Can you work these out from the model? Positions are in its coordinate system, mm. A direction names the side the tool comes from. Round coordinates to 2 decimals unless told otherwise and drop trailing zeros. Loops run counter-clockwise (first coordinate to the right, second up) from the corner with the lowest first, then second, coordinate; pieces in that order, holes last.
(1) Will these pins go through, and if not, where does the flat tip stop? pin 1 Ø3 at (y, z) = (20.48, 18.5) entering from +X; pin 2 Ø8 at (x, y) = (16, -20) entering from +Z; pin 3 Ø6 at (x, y) = (-9.5, 18) entering from -Z; pin 4 Ø5 at (x, z) = (75, 31) entering from +Y.
(2) Which directions (+Z, -Z, +X, -X, +Y, -Y) give clear straight access to the entire face, cutting with the end or side of a thin tool? Please do faces 5 (the face through (-105, -6, 30)), 6 (the face through (1, -3, 13.5)), 7 (the face through (-109, -9, 21)).
(3) Thinking about a two-plate mould opening in Y: for faces 1 (the face through (-103, -9, 19)), 2 (the face through (103.289, 24.778, 6.844)), 3 (the face through (1, 30, 37)), 4 (the face through (-110.07, -21.896, 32.819)), which applies, released by +Y, released by -Y, zero draft, split by the parting line, or undercut?
(4) I want a section at A-A on x = -75. Write out the boundary of the cut face in (y, z).
(5) If I drill on line 1 along X through (y, z) = (15, 11); line 2 along Y through (x, z) = (-68, 4); line 3 along Z through (x, y) = (31.5, -19), over which ranges is the centre line in solid material (lowest first)?
(6) I want a section at C-C on x = 89. Write out the boundary of the cut face in (y, z), plus the area to 3 significant figures.
(7) I want a section at B-B on y = 8.5. Write out the boundary of the cut face in (x, z), plus the area to 3 significant figures.
from build123d import *

# Parameters (mm, degrees)
F0_W     = 115
F0_H     = 70
F1_DEPTH = 37
F2_R     = 2.75
F2_R_2   = 2.5
F3_DEPTH = 12
F4_W     = 105
F4_H     = 13.5
F5_DEPTH = 58
F6_R     = 3
F7_DEPTH = 70.001
F9_R     = 6


with BuildPart() as f1:
    # F0 (on Top) → F1 (new body)
    with BuildSketch(Plane.XY):
        with Locations((-57.5, 3.58214689)):
            Rectangle(F0_W, F0_H)
    extrude(amount=F1_DEPTH)

    # F2 (on face) → F3 (cut)
    with BuildSketch(Plane(origin=(-115, 0, 0), x_dir=(0, -1, 0), z_dir=(-1, 0, 0))):
        with Locations((-14.58214689, 30.5)):
            Circle(F2_R)
        with Locations((-14.58214689, 6.5)):
            Circle(F2_R)
        with Locations((20.41785311, 6.5)):
            Circle(F2_R)
        with Locations((20.41785311, 30.5)):
            Circle(F2_R)
        with Locations((-20.48214689, 18.5)):
            Circle(F2_R_2)
        with Locations((9.01785311, 18.5)):
            Circle(F2_R_2)
    extrude(amount=-F3_DEPTH, mode=Mode.SUBTRACT)

    # F4 (on face) → F5 (cut)
    with BuildSketch(Plane.XZ.offset(31.41785311)):
        with Locations((-52.5, 6.75)):
            Rectangle(F4_W, F4_H)
        with Locations((-52.5, 30.25)):
            Rectangle(F4_W, F4_H)
    extrude(amount=-F5_DEPTH, mode=Mode.SUBTRACT)

    # F6 (on face) → F7 (cut, through all)
    with BuildSketch(Plane(origin=(0, 38.58214689, 0), x_dir=(-1, 0, 0), z_dir=(0, 1, 0))):
        with Locations((75, 6)):
            Circle(F6_R)
        with Locations((75, 31)):
            Circle(F6_R)
        with Locations((25, 31)):
            Circle(F6_R)
        with Locations((25, 6)):
            Circle(F6_R)
    extrude(amount=-F7_DEPTH, mode=Mode.SUBTRACT)

    # F8: F1 across plane


with BuildPart() as f1_1:
    add(f1.part)
    add(f1.part.mirror(Plane.YZ))

    # F9
    f9_edges = [f1_1.edges().sort_by_distance(p)[0] for p in [
        (-105, 26.582147, 6.75),
        (105, 26.582147, 6.75),
        (-105, 26.582147, 30.25),
        (105, 26.582147, 30.25),
    ]]
    fillet(f9_edges, radius=F9_R)


solid = f1_1.part
Filled sheet:
1. pin 1: stops at x = 103
1. pin 2: stops at z = 23.5
1. pin 3: stops at z = 13.5
1. pin 4: passes through
2. face 5: +Z, -Y
2. face 6: -Z, -Y
2. face 7: -X
3. face 1: undercut
3. face 2: released by -Y
3. face 3: zero draft
3. face 4: undercut
4. outline: (-31.42, 13.5) - (26.58, 13.5) - (26.58, 9) - (38.58, 9) - (38.58, 28) - (26.58, 28) - (26.58, 23.5) - (-31.42, 23.5) - close; (26.58, 0) - (38.58, 0) - (38.58, 3) - (26.58, 3) - close; (26.58, 34) - (38.58, 34) - (38.58, 37) - (26.58, 37) - close
5. line 1: x = -115 to -105, 105 to 115
5. line 2: y = 26.58 to 38.58
5. line 3: z = 13.5 to 23.5
6. outline: (-31.42, 13.5) - (26.58, 13.5) - (26.58, 0) - (38.58, 0) - (38.58, 37) - (26.58, 37) - (26.58, 23.5) - (-31.42, 23.5) - close
6. area: 1,020 mm2
7. outline: (-115, 0) - (-105, 0) - (-105, 13.5) - (105, 13.5) - (105, 0) - (115, 0) - (115, 37) - (105, 37) - (105, 23.5) - (-105, 23.5) - (-105, 37) - (-115, 37) - close
7. area: 2,840 mm2
